```python
from build123d import *

# Parameters (mm, degrees)
SKETCH3_W               = 262.8
SKETCH3_H               = 305.28
BOSS_EXTRUDE3_DEPTH     = 410
CUT_EXTRUDE1_DEPTH      = 457.798565672
CUT_EXTRUDE1_DEPTH_BACK = 457.798565672
CUT_EXTRUDE2_DEPTH      = 457.798565672
CUT_EXTRUDE2_DEPTH_BACK = 457.798565672
SKETCH5_R               = 36
SKETCH6_W               = 154.08
SKETCH6_H               = 154.08
BOSS_EXTRUDE4_DEPTH     = 10
SKETCH7_R               = 75
BOSS_EXTRUDE5_DEPTH     = 30


with BuildPart() as part:
    # Sketch3 → Boss-Extrude3 (new body)
    with BuildSketch(Plane(origin=(0, 0, 0), x_dir=(1, 0, 0), z_dir=(0, 1, 0))):
        Rectangle(SKETCH3_W, SKETCH3_H)
    extrude(amount=BOSS_EXTRUDE3_DEPTH)

    # Sketch4 → Cut-Extrude1 (cut, two sides: drawn at the far end of the back side and taken through both)
    with BuildSketch(Plane(origin=(0, 410, 0), x_dir=(1, 0, 0), z_dir=(0, 1, 0)).offset(-CUT_EXTRUDE1_DEPTH_BACK)):
        with BuildLine():
            Line((-131.4, -90), (-131.4, -152.64))
            Line((-131.4, -152.64), (-70.92, -152.64))
            ThreePointArc((-70.92, -152.64), (-107.755247271, -127.687824951), (-131.4, -90))
        make_face()
        with BuildLine():
            Line((83.16, -152.64), (131.4, -152.64))
            Line((131.4, -152.64), (131.4, -72.72))
            ThreePointArc((131.4, -72.72), (117.938305095, -119.113391364), (83.16, -152.64))
        make_face()
        with BuildLine():
            Line((-99.372734155, 121.287125755), (-67.345468311, 121.287125755))
            Line((-67.345468311, 121.287125755), (-48.15934209, 152.64))
            Line((-48.15934209, 152.64), (-131.4, 152.64))
            Line((-131.4, 152.64), (-131.4, 83.52))
            ThreePointArc((-131.4, 83.52), (-119.737831056, 106.093689962), (-99.372734155, 121.287125755))
        make_face()
        with BuildLine():
            Line((131.4, 83.52), (131.4, 152.64))
            Line((131.4, 152.64), (62.28, 152.64))
            ThreePointArc((62.28, 152.64), (109.286007047, 130.526007047), (131.4, 83.52))
        make_face()
    extrude(amount=CUT_EXTRUDE1_DEPTH + CUT_EXTRUDE1_DEPTH_BACK, mode=Mode.SUBTRACT)

    # Sketch5 → Cut-Extrude2 (cut, two sides: drawn at the far end of the back side and taken through both)
    with BuildSketch(Plane(origin=(0, 410, 0), x_dir=(1, 0, 0), z_dir=(0, 1, 0)).offset(-CUT_EXTRUDE2_DEPTH_BACK)):
        with Locations(Location((0, 0, 0), (0, 0, 270))):
            Circle(SKETCH5_R)
    extrude(amount=CUT_EXTRUDE2_DEPTH + CUT_EXTRUDE2_DEPTH_BACK, mode=Mode.SUBTRACT)

    # Sketch6 → Boss-Extrude4 (add)
    with BuildSketch(Plane.XY.offset(152.64)):
        with Locations((6.12, 205)):
            Rectangle(SKETCH6_W, SKETCH6_H)
    extrude(amount=BOSS_EXTRUDE4_DEPTH)

    # Sketch7 → Boss-Extrude5 (add)
    with BuildSketch(Plane.XY.offset(162.64)):
        with Locations((6.12, 205)):
            Circle(SKETCH7_R)
    extrude(amount=BOSS_EXTRUDE5_DEPTH)


solid = part.part
```
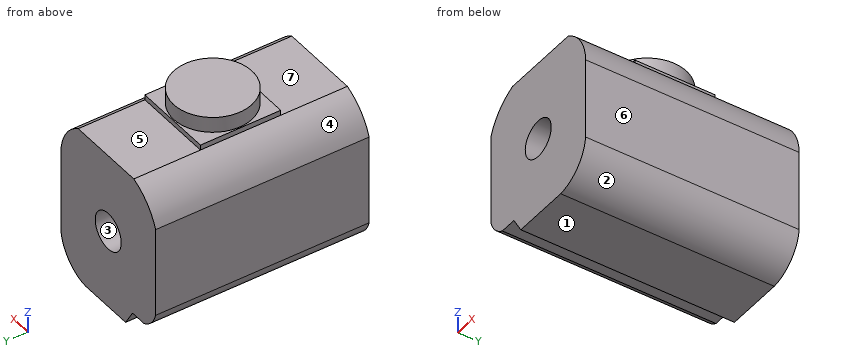
The listing builds one solid part. Answer for the finished solid, in the listing's coordinates (mm). Face numbers are marked on the shaded views. A direction names the side the tool comes from. Give positions to 0.01 mm unless a question says otherwise; leave off trailing zeros. Write each loop counter-clockwise with the first axis right and the second up, starting at its lowest first coordinate (ties: lowest second). Pieces come first, ordered by that corner, then holes. Notation, with made-up numbers: (-23.75, -11) - (29.25, -11) arc R22 ccw to (29.25, 12) - close; hole circle Ø2 at (1.25, 6). An arc over 180 degrees is marked (long way). Use one line per item in the form item = value. Start each with the question number.
1) Find section A-A on z = 0. Determine the outline of the cut face in (x, y), plus the area to 3 significant figures.
2) A tool of negligible diameter and unlimited length cuts with its end or side. For the marked faces 5, 6 and 7, from which of +Z, -Z, +X, -X, +Y, -Y can it reach the whole face along a straight path? Write none if from no direction.
3) Flat-ended cylindrical pins translate along their axes: pin 1 Ø8 at (x, y) = (72, 263) entering from +Z; pin 2 Ø2 at (x, y) = (29.5, 335) entering from +Z; pin 3 Ø5 at (x, y) = (-53.5, 236) entering from -Z. Find the tip coordinate at first contact, or state that the pin passes through.
4) The mould has two halves that part along X. Classify the marked faces 1, 2, 3 and 4: pulls with the +X half, pulls with the -X half, needs draft (parallel to the pull), parting line crosses it, or undercut.
5) Find section C-C on x = -24. Determine the outline of the cut face in (y, z).
6) Consider line 1 along Z through (x, y) = (0, 317); line 2 along X through (y, z) = (236, 0); line 3 along Z through (x, y) = (0, 229). Determine where each line is inside the solid, lowest interval first. Write a range as from..to.
7) Find section D-D on y = 195.5. Determine the outline of the cut face in (x, z), plus the area to 3 significant figures.
8) Find section B-B on y = 303.5. Determine the outline of the cut face in (x, z).
Geometry results:
q1.outline = (-131.4, 0) - (-36, 0) - (-36, 410) - (-131.4, 410) - close; (36, 0) - (131.4, 0) - (131.4, 410) - (36, 410) - close
q1.area = 78,200 mm2
q2.face_5 = +Z, +X, -X, +Y
q2.face_6 = +Z, -Z, +X, +Y, -Y
q2.face_7 = +Z, +X, -X, -Y
q3.pin_1 = 162.64
q3.pin_2 = 152.64
q3.pin_3 = -148
q4.face_1 = needs draft
q4.face_2 = pulls with the +X half
q4.face_3 = undercut
q4.face_4 = pulls with the -X half
q5.outline = (0, -152.64) - (410, -152.64) - (410, -26.83) - (0, -26.83) - close; (0, 26.83) - (410, 26.83) - (410, 152.64) - (282.04, 152.64) - (282.04, 162.64) - (273.69, 162.64) - (273.69, 192.64) - (136.31, 192.64) - (136.31, 162.64) - (127.96, 162.64) - (127.96, 152.64) - (0, 152.64) - close
q6.line_1 = -152.64..-36, 36..152.64
q6.line_2 = -131.4..-36, 36..131.4
q6.line_3 = -152.64..-36, 36..192.64
q7.outline = (-131.4, -83.52) arc R56.58 ccw to (-99.37, -121.29) - (-67.35, -121.29) - (-48.16, -152.64) - (62.28, -152.64) arc R76.66 ccw to (131.4, -83.52) - (131.4, 72.72) arc R93.72 ccw to (83.16, 152.64) - (83.16, 162.64) - (80.52, 162.64) - (80.52, 192.64) - (-68.28, 192.64) - (-68.28, 162.64) - (-70.92, 162.64) - (-70.92, 152.64) arc R107.96 ccw to (-131.4, 90) - close; hole circle Ø72 at (0, 0)
q7.area = 75,700 mm2
q8.outline = (-131.4, -83.52) arc R56.58 ccw to (-99.37, -121.29) - (-67.35, -121.29) - (-48.16, -152.64) - (62.28, -152.64) arc R76.66 ccw to (131.4, -83.52) - (131.4, 72.72) arc R93.72 ccw to (83.16, 152.64) - (-70.92, 152.64) arc R107.96 ccw to (-131.4, 90) - close; hole circle Ø72 at (0, 0)
